```python
from build123d import *

# Parameters (mm, degrees)
F1_DEPTH = 63.5
F0_W     = 13.734161
F0_H     = 19.05
F2_DEPTH = 25.4
F3_DEPTH = 7.9375
F0_W_2   = 25.4
F0_H_2   = 28.575
F5_R     = 6.35


with BuildPart() as f1:
    # F0 (on Front) → F1 (new body, symmetric)
    with BuildSketch(Plane.XZ):
        Polygon((36.758158, 16.938625), (-26.741842, 16.938625), (-26.741842, -2.111375), (55.808158, -2.111375), (55.808158, 16.938625), align=None)
    extrude(amount=F1_DEPTH, both=True)

    # F0 (on Front) → F2 (join, symmetric)
    with BuildSketch(Plane.XZ):
        with BuildLine():
            Line((36.758158, 34.337625), (36.758158, 16.938625))
            Line((36.758158, 16.938625), (55.808158, 16.938625))
            Line((55.808158, 16.938625), (55.808158, 34.337625))
            ThreePointArc((55.808158, 34.337625), (60.457838, 45.562945), (71.683158, 50.212625))
            Line((71.683158, 50.212625), (82.213558, 50.212625))
            Line((82.213558, 50.212625), (82.213558, 69.262625))
            Line((82.213558, 69.262625), (71.683158, 69.262625))
            add(Edge.make_bspline(
                [(71.332357, 69.260863), (71.449649, 69.261426), (71.566584, 69.262012), (71.683158, 69.262625)],
                knots=[111.087067, 111.087067, 111.087067, 111.087067, 111.468747, 111.468747, 111.468747, 111.468747], degree=3))
            ThreePointArc((71.332357, 69.260863), (46.863737, 58.908989), (36.758158, 34.337625))
        make_face()
        with Locations((89.080638, 59.737625)):
            Rectangle(F0_W, F0_H)
    extrude(amount=F2_DEPTH, both=True)

    # F0 (on Front) → F3 (join, symmetric)
    with BuildSketch(Plane.XZ):
        with BuildLine():
            add(Edge.make_bspline(
                [(-26.741842, 16.938625), (-27.171182, 70.95094), (37.19487, 69.097097), (71.332357, 69.260863)],
                knots=[0, 0, 0, 0, 111.087067, 111.087067, 111.087067, 111.087067], degree=3))
            Line((-26.741842, 16.938625), (36.758158, 16.938625))
            Line((36.758158, 16.938625), (36.758158, 34.337625))
            ThreePointArc((36.758158, 34.337625), (46.863737, 58.908989), (71.332357, 69.260863))
        make_face()
    extrude(amount=F3_DEPTH, both=True)

    # F0 (on Front) → F4 (revolve)
    with BuildSketch(Plane.XZ):
        with Locations((120.313558, 59.801125)):
            Rectangle(F0_W_2, F0_H_2)
    revolve(axis=Axis((107.613558, 0, 59.801125), (0, 0, -1)))

    # F5
    f5_edges = [f1.edges().sort_by_distance(p)[0] for p in [
        (-26.741842, -63.5, 7.413625),
        (55.808158, -63.5, 7.413625),
        (55.808158, 63.5, 7.413625),
        (-26.741842, 63.5, 7.413625),
    ]]
    fillet(f5_edges, radius=F5_R)


solid = f1.part
```
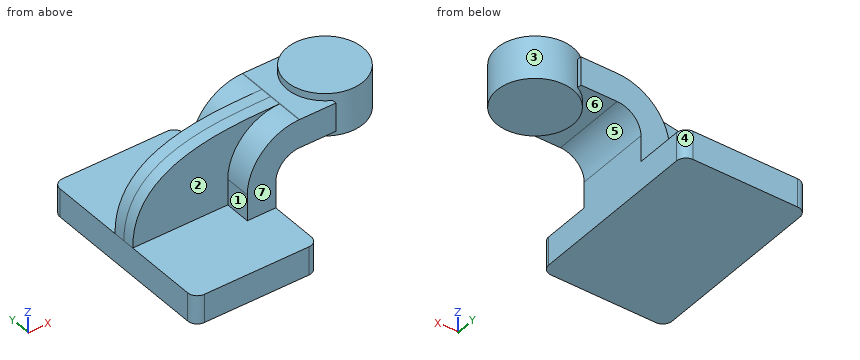
Geometry check sheet. Reference: the model listing, model coordinates, mm. Face numbers are marked on the shaded views. A direction names the side the tool comes from. Round coordinates to 2 decimals unless told otherwise and drop trailing zeros. Order: outer loops, then holes, each group sorted by start corner. A loop starts at its lowest first (then second) coordinate and runs counter-clockwise, first axis right, second up. Notation, with made-up numbers: (59.5, 70.25) -> (117.5, 70.25) arc R16 ccw to (117.5, 84.25) -> close; hole circle Ø9 at (43.25, 62.25). An arc over 180 degrees is marked (long way). Return JSON: item names as keys, results as strings. Group by question number.
Q1. Release check for a two-part mould opening along X. For the marked faces 1, 2, 3 and 4 record: released by +X, released by -X, zero draft, split by the parting line, or undercut.
Q2. Section check A-A, the plane z = 13.5. Record the boundary of the cut face in (x, y).
Q3. Section check C-C, the plane x = 117. Record the boundary of the cut face in (y, z), plus the area to 3 significant figures.
Q4. Gauge pin test, flat ends, axial feed: pin 1 (1.4 mm diameter, centred on y = 24, z = 59, fed in from +X); pin 2 (0.9 mm diameter, centred on y = -23.5, z = 63.5, fed in from +X); pin 3 (19 mm diameter, centred on y = -18.5, z = 22.5, fed in from -X). Record the tip position at first contact, or that the pin passes through.
Q5. Section check B-B, the plane y = 34. Record the boundary of the cut face in (x, z).
Q6. Material ranges on probe 1 along Y at (x, z) = (4, 30); probe 2 along Y at (x, z) = (68, 55.5); probe 3 along X at (y, z) = (-8, 49), recorded low to high. Write a range as from..to.
Q7. Tool access check on the marked faces 5, 6 and 7. Record the directions out of +Z, -Z, +X, -X, +Y, -Y that give a thin tool (end or side, any length) a straight path to the whole face; none if there is none.
Numbers:
{
 "1": {"face 1": "released by -X", "face 2": "zero draft", "face 3": "undercut", "face 4": "released by +X"},
 "2": {"outline": "(-26.74, -57.15) arc R6.35 ccw to (-20.39, -63.5) -> (49.46, -63.5) arc R6.35 ccw to (55.81, -57.15) -> (55.81, 57.15) arc R6.35 ccw to (49.46, 63.5) -> (-20.39, 63.5) arc R6.35 ccw to (-26.74, 57.15) -> close"},
 "3": {"outline": "(-23.6, 45.51) -> (23.6, 45.51) -> (23.6, 74.09) -> (-23.6, 74.09) -> close", "area": "1,350 mm^2"},
 "4": {"pin 1": "x = 117.73", "pin 2": "x = 118.28", "pin 3": "x = -26.74"},
 "5": {"outline": "(-26.74, -2.11) -> (55.81, -2.11) -> (55.81, 16.94) -> (-26.74, 16.94) -> close"},
 "6": {"probe 1": "-7.94..7.94", "probe 2": "-25.4..25.4", "probe 3": "39.99..65.6, 83.51..131.72"},
 "7": {"face 5": "-Z, +Y, -Y", "face 6": "-Z", "face 7": "+Z, +X, -X, -Y"}
}
